The drawing under review shows one solid part. Ordinate dimensions are in mm from its lowest x, y, z. Round coordinates to 2 decimals unless told otherwise and drop trailing zeros. Order: outer loops, then holes, each group sorted by start corner. A loop starts at its lowest first (then second) coordinate and runs counter-clockwise, first axis right, second up. Notation, with made-up numbers: M 37,45 L 79,45 A6 cw 79,51 Z; hole C -30,59.25 d6. An arc over 180 degrees is marked long. Answer as a JSON object with one key per item and string values.
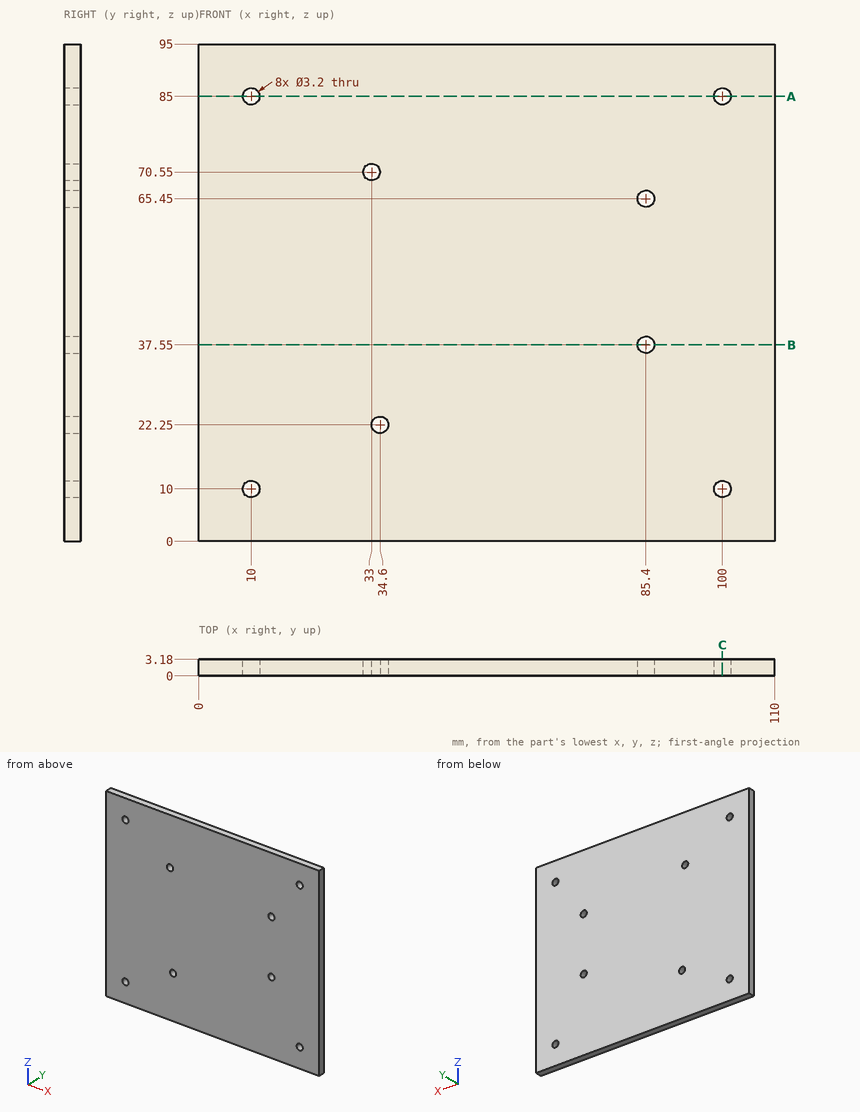
1) Add section A-A on z = 85. State the section outline as (x, y) points.
Geometry check:
{"outline": "M 0,0 L 8.4,0 L 8.4,3.18 L 0,3.18 Z; M 11.6,0 L 98.4,0 L 98.4,3.18 L 11.6,3.18 Z; M 101.6,0 L 110,0 L 110,3.18 L 101.6,3.18 Z"}
2) For L1, parallel to Z at x = 10, y = 1.5; L2, parallel to Z at x = 85.4, y = 0.7; L3, parallel to X at y = 1.3, z = 10, list the stretches that pass through material, from the lowest coordinate up.
Geometry check:
{"L1": "z = 0 to 8.4, 11.6 to 83.4, 86.6 to 95", "L2": "z = 0 to 35.95, 39.15 to 63.85, 67.05 to 95", "L3": "x = 0 to 8.4, 11.6 to 98.4, 101.6 to 110"}
3) Add section C-C on x = 100. State the section outline as (y, z) points, and give its area (3 significant figures).
Geometry check:
{"outline": "M 0,0 L 3.18,0 L 3.18,8.4 L 0,8.4 Z; M 0,11.6 L 3.18,11.6 L 3.18,83.4 L 0,83.4 Z; M 0,86.6 L 3.18,86.6 L 3.18,95 L 0,95 Z", "area": "282 mm²"}
4) Add section B-B on z = 37.55. State the section outline as (x, y) points.
Geometry check:
{"outline": "M 0,0 L 83.8,0 L 83.8,3.18 L 0,3.18 Z; M 87,0 L 110,0 L 110,3.18 L 87,3.18 Z"}
